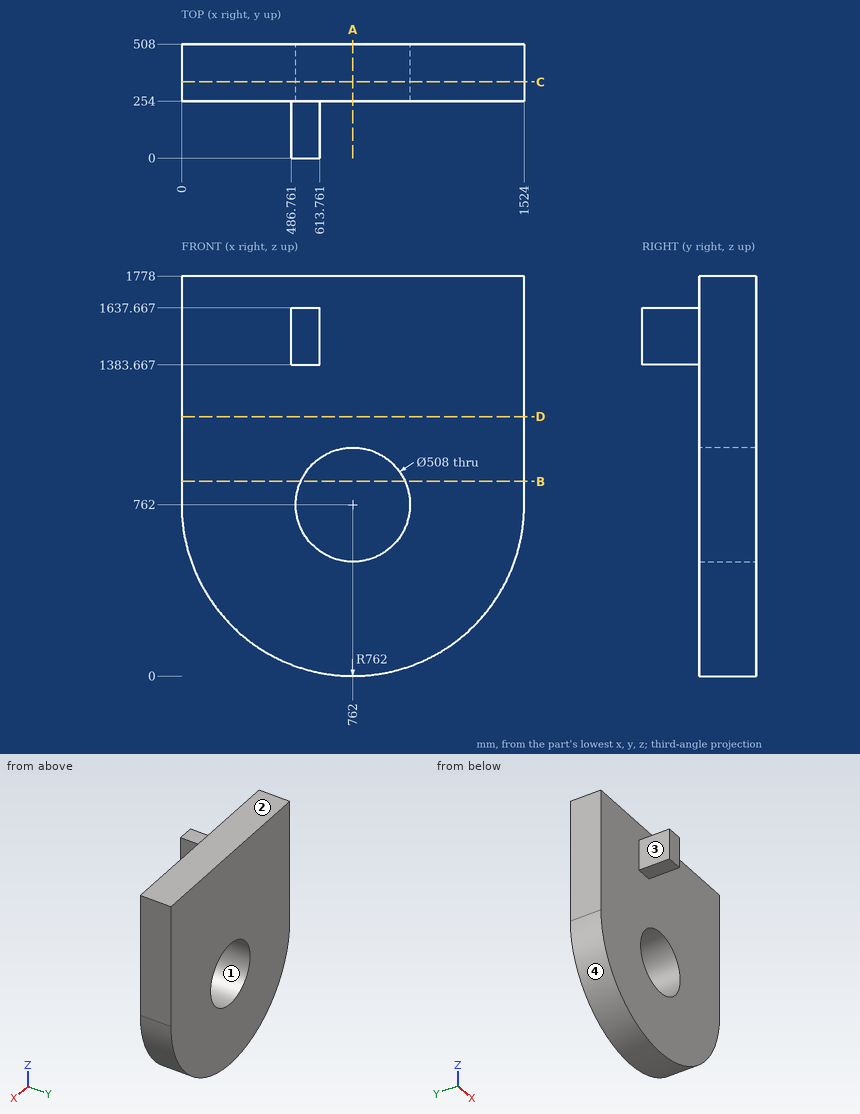
Design review of the part shown in the three views and the two pictorial views. Dimensions are in mm from the part's minimum x, y and z. Round coordinates to 2 decimals unless told otherwise and drop trailing zeros. Loops run counter-clockwise (first coordinate to the right, second up) from the corner with the lowest first, then second, coordinate; pieces in that order, holes last.
(1) Mouldability with a two-part tool opening along Z and no side actions: class the marked faces 1, 2, 3 and 4 as released by +Z, released by -Z, zero draft, split by the parting line, or undercut.
Returned:
face 1: undercut
face 2: released by +Z
face 3: zero draft
face 4: released by -Z
(2) We need section C-C (y = 339). Give the boundary of the cut face in (x, z), plus the area to 3 significant figures.
Returned:
outline: (0, 762) arc R762 ccw to (1524, 762) - (1524, 1778) - (0, 1778) - close; hole circle Ø508 at (762, 762)
area: 2,260,000 mm2
(3) We need section A-A (x = 762). Give the boundary of the cut face in (y, z), plus the area to 3 significant figures.
Returned:
outline: (254, 0) - (508, 0) - (508, 508) - (254, 508) - close; (254, 1016) - (508, 1016) - (508, 1778) - (254, 1778) - close
area: 323,000 mm2
(4) We need section D-D (z = 1154). Give the boundary of the cut face in (x, y), plus the area to 3 significant figures.
Returned:
outline: (0, 254) - (1524, 254) - (1524, 508) - (0, 508) - close
area: 387,000 mm2
(5) Clearance check with flat-ended pins moving along their axes: P1, Ø10, axis at y = 435, z = 461, coming from the +X side; P2, Ø5, axis at y = 343.5, z = 1295.5, coming from the -X side. State where each tip first meets the part, or that it passes through.
Returned:
P1: stops at x = 1464.16
P2: stops at x = 0
(6) We need section B-B (z = 866). Give the boundary of the cut face in (x, y).
Returned:
outline: (0, 254) - (530.27, 254) - (530.27, 508) - (0, 508) - close; (993.73, 254) - (1524, 254) - (1524, 508) - (993.73, 508) - close
(7) Wall thickness on line 1 along X through (y, z) = (367, 762); line 2 along Y through (x, z) = (1017, 78); line 3 along X through (y, z) = (273, 153.5): over which ranges is each line inside the solid? List them lowest first.
Returned:
line 1: x = 0 to 508, 1016 to 1524
line 2: y = 254 to 508
line 3: x = 303.34 to 1220.66
